The listing builds one solid part. Answer for the finished solid, in the listing's coordinates (mm). Face numbers are marked on the shaded views. A direction names the side the tool comes from. Give positions to 0.01 mm unless a question says otherwise; leave off trailing zeros. Loops run counter-clockwise (first coordinate to the right, second up) from the corner with the lowest first, then second, coordinate; pieces in that order, holes last. Notation, with made-up numbers: M 70,32.25 L 88,32.25 A18 cw 88,48.25 Z; hole C -16,-5 d2. An arc over 180 degrees is marked long. Return JSON: item names as keys, results as strings.
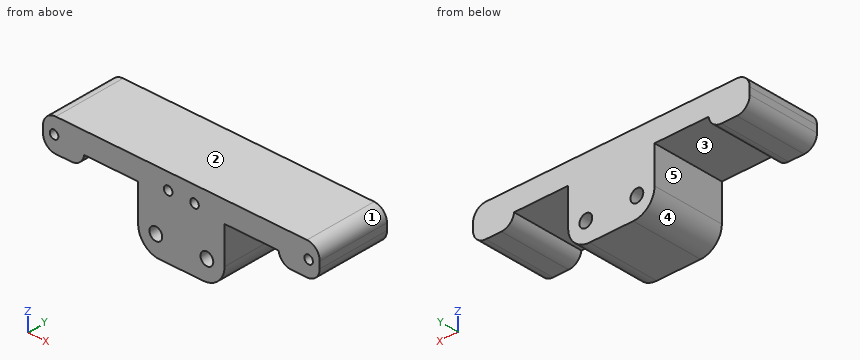
from build123d import *

# Parameters (mm, degrees)
SKETCH1_R           = 1.5
BOSS_EXTRUDE1_DEPTH = 17
SKETCH2_R           = 1
CUT_EXTRUDE1_DEPTH  = 12
FILLET2_R           = 5
FILLET3_R           = 3


with BuildPart() as part:
    # Sketch1 → Boss-Extrude1 (new body)
    with BuildSketch(Plane(origin=(0, 0, 0), x_dir=(1, 0, 0), z_dir=(0, 1, 0))):
        Polygon((-32.5, -13.8), (32.5, -13.8), (32.5, -6.2), (22.85, -6.2), (22.85, -8.84), (10.15, -8.84), (10.15, -6.2), (10.15, 4.8), (-10.15, 4.8), (-10.15, -8.84), (-22.85, -8.84), (-22.85, -6.2), (-32.5, -6.2), align=None)
        with Locations(Location((-6, 0, 0), (0, 0, 270))):
            Circle(SKETCH1_R, mode=Mode.SUBTRACT)
        with Locations(Location((6, 0, 0), (0, 0, 270))):
            Circle(SKETCH1_R, mode=Mode.SUBTRACT)
    extrude(amount=BOSS_EXTRUDE1_DEPTH)

    # Sketch2 → Cut-Extrude1 (cut)
    with BuildSketch(Plane.XZ):
        with Locations(Location((-3.1, 10, 0), (0, 0, 270))):
            Circle(SKETCH2_R)
        with Locations(Location((-29.9, 10, 0), (0, 0, 270))):
            Circle(SKETCH2_R)
        with Locations(Location((3.1, 10, 0), (0, 0, 270))):
            Circle(SKETCH2_R)
        with Locations(Location((29.9, 10, 0), (0, 0, 270))):
            Circle(SKETCH2_R)
    extrude(amount=-CUT_EXTRUDE1_DEPTH, mode=Mode.SUBTRACT)

    # Fillet2
    fillet2_edges = [part.edges().sort_by_distance(p)[0] for p in [
        (-10.15, 8.5, -4.8),
        (10.15, 8.5, -4.8),
    ]]
    fillet(fillet2_edges, radius=FILLET2_R)

    # Fillet3
    # the kernel refuses this fillet: 3 mm, written as the material it takes off along each edge
    with BuildSketch(Plane(origin=(-32.5, -7.5, 13.8), x_dir=(0, 0, -1), z_dir=(0, 1, 0)), Plane(origin=(32.5, -7.5, 13.8), x_dir=(-1, 0, 0), z_dir=(0, 1, 0)), Plane(origin=(32.5, -7.5, 6.2), x_dir=(0, 0, 1), z_dir=(0, 1, 0)), Plane(origin=(-32.5, -7.5, 6.2), x_dir=(1, 0, 0), z_dir=(0, 1, 0))) as fillet3_piece_1:
        with BuildLine():
            CenterArc((FILLET3_R, -FILLET3_R), FILLET3_R, 90, 90)
            Line((0, -FILLET3_R), (-FILLET3_R * 0.02, -FILLET3_R))
            Line((-FILLET3_R * 0.02, -FILLET3_R), (-FILLET3_R * 0.02, FILLET3_R * 0.02))
            Line((-FILLET3_R * 0.02, FILLET3_R * 0.02), (FILLET3_R, FILLET3_R * 0.02))
            Line((FILLET3_R, FILLET3_R * 0.02), (FILLET3_R, 0))
        make_face()
    extrude(amount=32, mode=Mode.SUBTRACT)
    with BuildSketch(Plane(origin=(22.85, -7.445804188, 6.2), x_dir=(0, 0, 1), z_dir=(0, 1, 0))) as fillet3_piece_2:
        with BuildLine():
            CenterArc((3, 2.978321675), FILLET3_R, 180, 83.107897421)
            Line((0, 2.978321675), (-0.06, 2.978321675))
            Line((-0.06, 2.978321675), (-0.06, 0))
            Line((-0.06, 0), (0, -0.06))
            ThreePointArc((0, -0.06), (1.32, -0.06), (2.6328, -0.059566434))
            Line((2.6328, -0.059566434), (2.64, 0))
        make_face()
    extrude(amount=31.891608375, mode=Mode.SUBTRACT)
    with BuildSketch(Plane(origin=(-22.85, -7.445804188, 6.2), x_dir=(0, 0, 1), z_dir=(0, 1, 0))) as fillet3_piece_3:
        with BuildLine():
            CenterArc((3, -2.978321675), FILLET3_R, 96.892102579, 83.107897421)
            Line((0, -2.978321675), (-0.06, -2.978321675))
            Line((-0.06, -2.978321675), (-0.06, 0))
            Line((-0.06, 0), (0, 0.06))
            ThreePointArc((0, 0.06), (1.32, 0.06), (2.6328, 0.059566434))
            Line((2.6328, 0.059566434), (2.64, 0))
        make_face()
    extrude(amount=31.891608375, mode=Mode.SUBTRACT)


solid = part.part
(1) A tool of negligible diameter and unlimited length cuts with its end or side. For the marked faces 4 and 5, from which of +Z, -Z, +X, -X, +Y, -Y can it reach the whole face along a straight path? Write none if from no direction.
Values follow:
{"face 4": "-Z, -X, +Y, -Y", "face 5": "-Z, +Y, -Y"}
(2) The part is cut by section C-C (x = 3.1). Determine the outline of the cut face in (y, z), and give its area (3 significant figures).
Values follow:
{"outline": "M 0,-4.8 L 17,-4.8 L 17,13.8 L 0,13.8 L 0,11 L 12,11 L 12,9 L 0,9 Z", "area": "292 mm²"}
(3) The part is cut by section B-B (y = 5.5). Determine the outline of the cut face in (x, z).
Values follow:
{"outline": "M -32.5,9.2 A3 ccw -29.5,6.2 L -25.83,6.2 A3 ccw -22.85,8.84 L -10.15,8.84 L -10.15,0.2 A5 ccw -5.15,-4.8 L 5.15,-4.8 A5 ccw 10.15,0.2 L 10.15,8.84 L 22.85,8.84 A3 ccw 25.83,6.2 L 29.5,6.2 A3 ccw 32.5,9.2 L 32.5,10.8 A3 ccw 29.5,13.8 L -29.5,13.8 A3 ccw -32.5,10.8 Z; hole C -29.9,10 d2; hole C -6,0 d3; hole C -3.1,10 d2; hole C 3.1,10 d2; hole C 6,0 d3; hole C 29.9,10 d2"}
(4) Determine the mould class of the marked faces 1, 2 and 3 for opening direction X: released by +X, released by -X, zero draft, split by the parting line, or undercut.
Values follow:
{"face 1": "released by +X", "face 2": "zero draft", "face 3": "undercut"}
(5) The part is cut by section A-A (y = 14.25). Determine the outline of the cut face in (x, z).
Values follow:
{"outline": "M -32.5,9.2 A3 ccw -29.5,6.2 L -25.83,6.2 A3 ccw -22.85,8.84 L -10.15,8.84 L -10.15,0.2 A5 ccw -5.15,-4.8 L 5.15,-4.8 A5 ccw 10.15,0.2 L 10.15,8.84 L 22.85,8.84 A3 ccw 25.83,6.2 L 29.5,6.2 A3 ccw 32.5,9.2 L 32.5,10.8 A3 ccw 29.5,13.8 L -29.5,13.8 A3 ccw -32.5,10.8 Z; hole C -6,0 d3; hole C 6,0 d3"}
(6) Straight lines are drawn through the part: line 1 along X through (y, z) = (11.5, 0); line 2 along X through (y, z) = (6.25, 10); line 3 along Z through (x, y) = (17.5, 13.5). For each, find the intervals that lie inside material, in ascending order.
Values follow:
{"line 1": "-10.15 to -7.5, -4.5 to 4.5, 7.5 to 10.15", "line 2": "-32.5 to -30.9, -28.9 to -4.1, -2.1 to 2.1, 4.1 to 28.9, 30.9 to 32.5", "line 3": "8.84 to 13.8"}
(7) Given pin 1 (2 mm diameter, centred on x = -18.5, y = 4, fed in from -Z); pin 2 (2.5 mm diameter, centred on x = 6, z = 0, fed in from +Y); pin 3 (0.6 mm diameter, centred on x = 3, z = 10, fed in from -Y); pin 4 (1.5 mm diameter, centred on y = 8.5, z = 7, fed in from -X), each flat-ended and moving along its own axis, determine where each tip first touches the part or whether it passes through.
Values follow:
{"pin 1": "z = 8.84", "pin 2": "through", "pin 3": "y = 12", "pin 4": "x = -32.13"}
(8) The part is cut by section D-D (z = 10). Determine the outline of the cut face in (x, y).
Values follow:
{"outline": "M -32.5,0 L -30.9,0 L -30.9,12 L -28.9,12 L -28.9,0 L -4.1,0 L -4.1,12 L -2.1,12 L -2.1,0 L 2.1,0 L 2.1,12 L 4.1,12 L 4.1,0 L 28.9,0 L 28.9,12 L 30.9,12 L 30.9,0 L 32.5,0 L 32.5,17 L -32.5,17 Z"}
